Part model, mm, in its own coordinate system. A direction names the side the tool comes from. Round coordinates to 2 decimals unless told otherwise and drop trailing zeros. Answer as CSV lines item,"result". Start each with the question number.
Item 1: Mould opens along X. For faces 3 (the flat face through (-1, 96.8, -3)), 4 (the conical face through (-48.111, -79.478, 2.393)), 5 (the flat face through (-55.8, -1, -3)), 6 (the conical face through (48.111, 79.478, 2.393)) say: pulls with the +X half, pulls with the -X half, needs draft (parallel to the pull), parting line crosses it, or undercut.
Item 2: Which spindle directions (+Z, -Z, +X, -X, +Y, -Y) get a long thin tool onto all of the face, cutting with end or side? Do faces 1 (the cylindrical face through (-52.718, -93.605, -2.958)), 2 (the flat face through (1, -96.8, -3)). Say none if no direction does.
Item 3: Drop flat-ended pins along their axis: pin 1 Ø1.8 at (x, z) = (-9, -3.5) entering from +Y; pin 2 Ø6 at (y, z) = (4, -5) entering from +X; pin 3 Ø1.6 at (x, z) = (-52.5, -3) entering from +Y. Give the stop position or say it passes through.
Item 4: Wall check: line 1 (Y direction, x = -30, z = -2.85); line 2 (Y direction, x = -46, z = -4.2); line 3 (X direction, y = -93.8, z = -2.35). Give the ranges that are in metal, low to high.
Autodesk Inventor part; units mm, degrees
ref_plane "Work Plane3" through (-58.9, -99.9, 0) normal (0, 0, 1) x (1, 0, 0)
ref_plane "Work Plane4" through (-51.1175, -82.55, -7.874) normal (0, 0, -1) x (0, 1, 0)
ref_plane "YZ Plane" through (0, 0, 0) normal (1, 0, 0) x (0, 1, 0)
ref_plane "Work Plane1" through (0, 0, 2.9972) normal (0, 0, 1) x (1, 0, 0)
ref_plane "Work Plane3" through (-58.9, -99.9, 0) normal (0, 0, 1) x (1, 0, 0)
sketch "Sketch2" plane through (0, 0, 2.9972) normal (0, 0, 1) x (1, 0, 0)
  line L0 (51.1175, 82.55) -> (51.1175, -82.55) construction
  line L1 (-51.1175, 82.55) -> (51.1175, 82.55) construction
  line L2 (-51.1175, -82.55) -> (-51.1175, 82.55) construction
  line L3 (51.1175, -82.55) -> (-51.1175, -82.55) construction
  arc A0 (58.9, 88.5) -> (47.5, 99.9) centre (47.5, 88.5) ccw
  line L4 (47.5, 99.9) -> (-47.5, 99.9)
  line L5 (58.9, -88.5) -> (58.9, 88.5)
  arc A1 (47.5, -99.9) -> (58.9, -88.5) centre (47.5, -88.5) ccw
  line L6 (-47.5, -99.9) -> (47.5, -99.9)
  arc A2 (-58.9, -88.5) -> (-47.5, -99.9) centre (-47.5, -88.5) ccw
  line L7 (-58.9, 88.5) -> (-58.9, -88.5)
  arc A3 (-47.5, 99.9) -> (-58.9, 88.5) centre (-47.5, 88.5) ccw
  line L8 (48.1175, -79.55) -> (48.1175, 79.55)
  line L9 (48.1175, 79.55) -> (-48.1175, 79.55)
  line L10 (-48.1175, 79.55) -> (-48.1175, -79.55)
  line L11 (-48.1175, -79.55) -> (48.1175, -79.55)
  point P0 (0, 0)
  dimension "d1" = 3
extrude "Extrusion1" add sketch "Sketch2" against normal up to surface (2.9972 mm away)
fillet "Fillet1" radius 3 4 edges at (48.1175, 79.55, 1.4986) (48.1175, -79.55, 1.4986) (-48.1175, -79.55, 1.4986) (-48.1175, 79.55, 1.4986)
chamfer "Chamfer1" distance 3 distance2 1 4 edges at (48.1175, 0, 2.9972) (0, -79.55, 2.9972) (-48.1175, 0, 2.9972) (0, 79.55, 2.9972) measured on face at (15.0392, -93.1167, 2.9972)
sketch "Sketch3" plane through (47.5, 99.9, 0) normal (0, 0, -1) x (-1, 0, 0)
  line L0 (98.6175, -17.35) -> (-3.6175, -17.35) construction
  line L1 (98.6175, -182.45) -> (98.6175, -17.35) construction
  line L2 (-3.6175, -182.45) -> (98.6175, -182.45) construction
  line L3 (-3.6175, -17.35) -> (-3.6175, -182.45) construction
  line L4 (95, -196.8) -> (0, -196.8) construction
  arc A0 (-8.4, -188.4) -> (0, -196.8) centre (0, -188.4) ccw construction
  line L5 (-8.4, -188.4) -> (-8.4, -11.4) construction
  arc A1 (0, -3) -> (-8.4, -11.4) centre (0, -11.4) ccw construction
  line L6 (0, -3) -> (95, -3) construction
  arc A2 (103.4, -11.4) -> (95, -3) centre (95, -11.4) ccw construction
  line L7 (103.4, -11.4) -> (103.4, -188.4) construction
  arc A3 (95, -196.8) -> (103.4, -188.4) centre (95, -188.4) ccw construction
  line L8 (-3.7175, -17.25) -> (98.7175, -17.25)
  line L9 (98.7175, -17.25) -> (98.7175, -182.55)
  line L10 (98.7175, -182.55) -> (-3.7175, -182.55)
  line L11 (-3.7175, -182.55) -> (-3.7175, -17.25)
  line L12 (95, -3.1) -> (0, -3.1)
  arc A4 (0, -3.1) -> (-8.3, -11.4) centre (0, -11.4) ccw
  line L13 (-8.3, -11.4) -> (-8.3, -188.4)
  arc A5 (-8.3, -188.4) -> (0, -196.7) centre (0, -188.4) ccw
  line L14 (0, -196.7) -> (95, -196.7)
  arc A6 (95, -196.7) -> (103.3, -188.4) centre (95, -188.4) ccw
  line L15 (103.3, -188.4) -> (103.3, -11.4)
  arc A7 (103.3, -11.4) -> (95, -3.1) centre (95, -11.4) ccw
  line L16 (100.7175, -15.25) -> (-5.7175, -15.25)
  line L17 (-5.7175, -15.25) -> (-5.7175, -184.55)
  line L18 (-5.7175, -184.55) -> (100.7175, -184.55)
  line L19 (100.7175, -184.55) -> (100.7175, -15.25)
  line L20 (100.7175, -172.55) -> (98.7175, -172.55)
  arc A8 (86.2825, -184.55) -> (100.7175, -184.55) centre (93.5, -184.55) ccw
  line L21 (86.2825, -184.55) -> (86.2825, -182.55)
  circle A9 centre (93.5, -177.4) radius 1.0065 construction
  line L22 (93.5, -177.4) -> (93.5, -184.55) construction
  point P0 (47.5, -99.9)
  dimension "d8" = 0.1
  dimension "d9" = 0.1
  dimension "d10" = 2
  dimension "d11" = 12
ref_plane "Work Plane4" through (-51.1175, -82.55, -7.874) normal (0, 0, -1) x (0, 1, 0)
extrude "Extrusion2" add sketch "Sketch3" along normal up to surface (7.874 mm away) contours L20 L19 L18 L21 L10 L9 | L18 A8
ref_plane "Work Plane5" through (0, -88.5, 2.9972) normal (1, 0, 0) x (0, 0, -1)
ref_plane "Work Plane6" through (-47.5, 0, 2.9972) normal (0, 1, 0) x (1, 0, 0)
sketch "Sketch5" plane through (-46, -84.65, -7.874) normal (0, 0, -1) x (-1, 0, 0)
  arc A0 (-7.2175, 0) -> (7.2175, 0) centre (0, 0) ccw
  line L0 (0, -7.2175) -> (0, 2) construction
  line L1 (-7.2175, 2) -> (5.2175, 2)
  point P0 (-46, 84.65)
  point P1 (0, -2.6087)
hole "Hole1" at (-46, -87.2587, -7.874) direction (0, 0, 1) diameter 3 depth 6 tip angle 118
mirror "Mirror1" about plane through (0, -88.5, 2.9972) normal (1, 0, 0) of "Extrusion2", "Hole1"
mirror "Mirror2" about plane through (-47.5, 0, 2.9972) normal (0, 1, 0) of "Extrusion2", "Hole1", "Mirror1"
fillet "Fillet2" radius 3 8 edges at (55.561, -96.561, 2.9972) (58.9, 0, 2.9972) (55.561, 96.561, 2.9972) (0, 99.9, 2.9972) (-55.561, 96.561, 2.9972) (-58.9, 0, 2.9972) (-55.561, -96.561, 2.9972) (0, -99.9, 2.9972)
sketch "Sketch6" plane through (47.5, 99.9, 0) normal (0, 0, -1) x (-1, 0, 0)
  line L0 (95, -196.8) -> (0, -196.8) construction
  line L1 (-8.4, -188.4) -> (-8.4, -11.4) construction
  line L2 (0, -3) -> (95, -3) construction
  line L3 (103.4, -11.4) -> (103.4, -188.4) construction
  arc A0 (-8.4, -188.4) -> (0, -196.8) centre (0, -188.4) ccw construction
  arc A1 (0, -3) -> (-8.4, -11.4) centre (0, -11.4) ccw construction
  arc A2 (103.4, -11.4) -> (95, -3) centre (95, -11.4) ccw construction
  arc A3 (95, -196.8) -> (103.4, -188.4) centre (95, -188.4) ccw construction
  line L4 (0, -196.7) -> (95, -196.7)
  arc A4 (95, -196.7) -> (103.3, -188.4) centre (95, -188.4) ccw
  line L5 (103.3, -188.4) -> (103.3, -11.4)
  arc A5 (103.3, -11.4) -> (95, -3.1) centre (95, -11.4) ccw
  line L6 (95, -3.1) -> (0, -3.1)
  arc A6 (0, -3.1) -> (-8.3, -11.4) centre (0, -11.4) ccw
  line L7 (-8.3, -11.4) -> (-8.3, -188.4)
  arc A7 (-8.3, -188.4) -> (0, -196.7) centre (0, -188.4) ccw
  line L8 (-7.3, -188.4) -> (-7.3, -11.4)
  arc A8 (0, -4.1) -> (-7.3, -11.4) centre (0, -11.4) ccw
  line L9 (0, -4.1) -> (95, -4.1)
  arc A9 (102.3, -11.4) -> (95, -4.1) centre (95, -11.4) ccw
  line L10 (102.3, -11.4) -> (102.3, -188.4)
  arc A10 (95, -195.7) -> (102.3, -188.4) centre (95, -188.4) ccw
  line L11 (95, -195.7) -> (0, -195.7)
  arc A11 (-7.3, -188.4) -> (0, -195.7) centre (0, -188.4) ccw
  arc A12 (23.5, -195.7) -> (11.5, -195.7) centre (17.5, -195.7) ccw
  line L12 (47.5, -195.7) -> (47.5, -4.1) construction
  arc A13 (83.5, -195.7) -> (71.5, -195.7) centre (77.5, -195.7) ccw
  line L13 (-7.3, -99.9) -> (102.3, -99.9) construction
  arc A14 (11.5, -4.1) -> (23.5, -4.1) centre (17.5, -4.1) ccw
  arc A15 (71.5, -4.1) -> (83.5, -4.1) centre (77.5, -4.1) ccw
  point P0 (47.5, -99.9)
  point P1 (11.5, -4.1)
  point P2 (23.5, -4.1)
  point P3 (83.5, -4.1)
  point P4 (83.5, -195.7)
  point P5 (71.5, -195.7)
  dimension "d22" = 0.1
  dimension "d23" = 1
  dimension "d24" = 6
  dimension "d34" = 60
extrude "Extrusion3" add sketch "Sketch6" along normal blind 6 contours A7 L7 A6 L6 A5 L5 A4 L4 | A12 L11 | L9 A14 | A13 L11 | L9 A15
sketch "Sketch8" plane through (47.5, 99.9, -6) normal (0, 0, -1) x (-1, 0, 0)
  line L0 (77.5, -6.1) -> (17.5, -6.1) construction
  line L1 (17.5, -6.1) -> (17.5, -193.7) construction
  line L2 (17.5, -193.7) -> (77.5, -193.7) construction
  line L3 (77.5, -193.7) -> (77.5, -6.1) construction
  line L4 (77.5, -6.1) -> (17.5, -193.7) construction
  line L5 (17.5, -6.1) -> (77.5, -193.7) construction
  line L6 (0, -196.7) -> (95, -196.7) construction
  point P0 (47.5, -99.9)
  dimension "d35" = 3
  dimension "d36" = 60
hole "Hole3" at (30, -93.8, -6) at (-30, -93.8, -6) at (-30, 93.8, -6) at (30, 93.8, -6) direction (0, 0, 1) diameter 3 depth 6 tip angle 118
properties part number "front-bezel"
Answer block:
1,face 3,"needs draft"
1,face 4,"undercut"
1,face 5,"pulls with the -X half"
1,face 6,"undercut"
2,face 1,"-Z"
2,face 2,"-Z, +X, -X, -Y"
3,pin 1,"stops at y = 96.8"
3,pin 2,"stops at x = 55.8"
3,pin 3,"stops at y = 95.66"
4,line 1,"y = -96.8 to -95.3, -92.3 to -89.8, 89.8 to 92.3, 95.3 to 96.8"
4,line 2,"y = -96.8 to -95.8, -91.87 to -88.76, -85.76 to -82.65, 82.65 to 85.76, 88.76 to 91.87, 95.8 to 96.8"
4,line 3,"x = -53.89 to -52.52, -35.66 to -31.5, -28.5 to -24.34, 24.34 to 28.5, 31.5 to 35.66, 52.52 to 53.89"
